Check sheet for the modelled part. Datum: model origin and axes. Units: mm. Face numbers are marked on the shaded views. Give positions to 0.01 mm unless a question says otherwise; leave off trailing zeros. Order: outer loops, then holes, each group sorted by start corner. A loop starts at its lowest first (then second) coordinate and runs counter-clockwise, first axis right, second up.
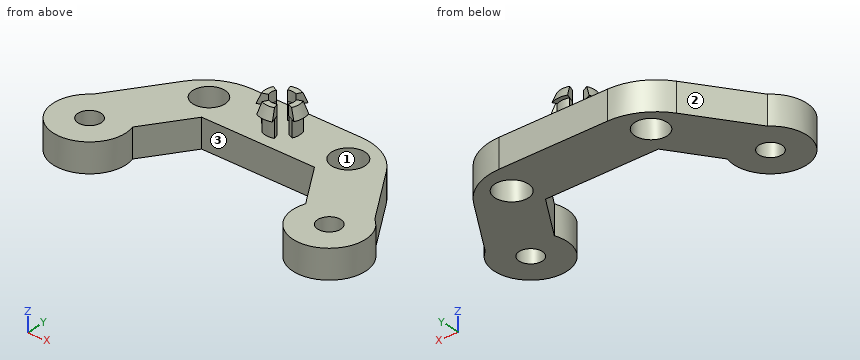
```python
from build123d import *

# Parameters (mm, degrees)
SZKIC1_R                    = 2
DODANIE_WYCI_GNI_CIE1_DEPTH = 5
SZKIC2_R                    = 2.797439786
SZKIC2_R_2                  = 2.890763472
WYTNIJ_WYCI_GNI_CIE1_DEPTH  = 10
ZAOKR_GLENIE1_R             = 10
DODANIE_WYCI_GNI_CIE2_DEPTH = 3
OBR_T1_ANGLE                = 45
SZYK_KO_OWY1_COUNT          = 4


# Read off the part's stored shape, not the designer's step: Obrót1
with BuildPart() as part:
    # Szkic1 → Dodanie-wyciągnięcie1 (new body)
    with BuildSketch(Plane.XY):
        with BuildLine():
            Line((-15, 0), (15, 0))
            Line((15, 0), (25, -15))
            ThreePointArc((25, -15), (23.099320571, -25.970135126), (15.330219835, -17.995329753))
            Line((15.330219835, -17.995329753), (10, -10))
            Line((10, -10), (-10, -10))
            Line((-10, -10), (-15.330219835, -17.995329753))
            ThreePointArc((-15.330219835, -17.995329753), (-23.099320571, -25.970135126), (-25, -15))
            Line((-25, -15), (-15, 0))
        make_face()
        with Locations((-21.25, -20)):
            Circle(SZKIC1_R, mode=Mode.SUBTRACT)
        with Locations((21.25, -20)):
            Circle(SZKIC1_R, mode=Mode.SUBTRACT)
    extrude(amount=DODANIE_WYCI_GNI_CIE1_DEPTH)

    # Szkic2 → Wytnij-wyciągnięcie1 (cut)
    with BuildSketch(Plane.XY.offset(5)):
        with Locations((-12.676758493, -5.398654495)):
            Circle(SZKIC2_R)
        with Locations((12.029040905, -5.398654495)):
            Circle(SZKIC2_R_2)
    extrude(amount=-WYTNIJ_WYCI_GNI_CIE1_DEPTH, mode=Mode.SUBTRACT)

    # Zaokrąglenie1
    zaokr_glenie1_edges = [part.edges().sort_by_distance(p)[0] for p in [
        (-15, 0, 2.5),
        (15, 0, 2.5),
    ]]
    fillet(zaokr_glenie1_edges, radius=ZAOKR_GLENIE1_R)

    # Szkic3 → Dodanie-wyciągnięcie2 (add)
    with BuildSketch(Plane.XY.offset(5)):
        with BuildLine():
            Line((-0.67948159, -3.118961784), (-1.019222385, -2.178442676))
            ThreePointArc((-1.019222385, -2.178442676), (0.136924764, -2.003126361), (1.272268294, -2.283139056))
            Line((1.272268294, -2.283139056), (0.848178863, -3.188759371))
            ThreePointArc((0.848178863, -3.188759371), (0.091283176, -3.002084241), (-0.67948159, -3.118961784))
        make_face()
        with BuildLine():
            Line((1.870588598, -4.292258312), (2.805882897, -3.938387468))
            ThreePointArc((2.805882897, -3.938387468), (2.999104941, -5.073277223), (2.750688951, -6.197376422))
            Line((2.750688951, -6.197376422), (1.833792634, -5.798250948))
            ThreePointArc((1.833792634, -5.798250948), (1.999403294, -5.048851482), (1.870588598, -4.292258312))
        make_face()
        with BuildLine():
            Line((0.692421598, -6.876313495), (1.038632398, -7.814470242))
            ThreePointArc((1.038632398, -7.814470242), (-0.113665121, -7.997845933), (-1.248768691, -7.727742062))
            Line((-1.248768691, -7.727742062), (-0.832512461, -6.818494708))
            ThreePointArc((-0.832512461, -6.818494708), (-0.075776747, -6.998563956), (0.692421598, -6.876313495))
        make_face()
        with BuildLine():
            Line((-1.884973157, -5.668487992), (-2.827459736, -6.002731988))
            ThreePointArc((-2.827459736, -6.002731988), (-2.996499858, -4.855125566), (-2.717538259, -3.72917908))
            Line((-2.717538259, -3.72917908), (-1.811692173, -4.152786053))
            ThreePointArc((-1.811692173, -4.152786053), (-1.997666572, -4.903417044), (-1.884973157, -5.668487992))
        make_face()
    extrude(amount=DODANIE_WYCI_GNI_CIE2_DEPTH)

    # Obrót1 outline → Obrót1 (revolve)
    with BuildSketch(Plane(origin=(0, -5, 0), x_dir=(0.42261826174070005, 0.9063077870366497, 0), z_dir=(0.9063077870366497, -0.42261826174070005, 0))):
        Polygon((3, 9.8), (2, 9.8), (2, 8), (3.781968342, 8), align=None)
    obr_t1 = revolve(axis=Axis((0, -5, 0), (0, 0, 1)), revolution_arc=OBR_T1_ANGLE)

    # Szyk kołowy1: Obrót1 ×4 about axis
    szyk_ko_owy1_axis = Axis((0, -5, 5), (0, 0, 1))
    for i in range(1, SZYK_KO_OWY1_COUNT):
        add(obr_t1.rotate(szyk_ko_owy1_axis, i * 360 / SZYK_KO_OWY1_COUNT))


solid = part.part
```
(1) Gauge pin test, flat ends, axial feed: pin 1 Ø10 at (x, y) = (18, -5.5) entering from +Z; pin 2 Ø4.5 at (x, y) = (12.03, -5.4) entering from -Z; pin 3 Ø1.5 at (y, z) = (-12, 3.5) entering from +X; pin 4 Ø5.5 at (x, z) = (2, 1.5) entering from -Y. Record the tip position at first contact, or that the pin passes through.
Response values:
pin 1: stops at z = 5
pin 2: passes through
pin 3: stops at x = 23.5
pin 4: stops at y = -10
(2) Cross-section at D-D on z = 2.5. Enter the section's corners in (x, y), then the cut area to 3 significant figures.
Response values:
outline: (-25, -15) arc R6.25 ccw (long way) to (-15.33, -18) - (-10, -10) - (10, -10) - (15.33, -18) arc R6.25 ccw (long way) to (25, -15) - (17.97, -4.45) arc R10 ccw to (9.65, 0) - (-9.65, 0) arc R10 ccw to (-17.97, -4.45) - close; hole circle Ø4 at (-21.25, -20); hole circle Ø5.59 at (-12.68, -5.4); hole circle Ø5.78 at (12.03, -5.4); hole circle Ø4 at (21.25, -20)
area: 642 mm2
(3) Cross-section at A-A on y = -20. Enter the section's corners in (x, z).
Response values:
outline: (-27.5, 0) - (-23.25, 0) - (-23.25, 5) - (-27.5, 5) - close; (-19.25, 0) - (-15, 0) - (-15, 5) - (-19.25, 5) - close; (15, 0) - (19.25, 0) - (19.25, 5) - (15, 5) - close; (23.25, 0) - (27.5, 0) - (27.5, 5) - (23.25, 5) - close
(4) Cross-section at B-B on x = 21. Enter the section's corners in (y, z) (3 decimals), then the cut area to 3 significant figures.
Response values:
outline: (-26.245, 0) - (-21.984, 0) - (-21.984, 5) - (-26.245, 5) - close; (-18.016, 0) - (-9, 0) - (-9, 5) - (-18.016, 5) - close
area: 66.4 mm2
(5) Release check for a two-part mould opening along Y. For the marked faces 1, 2 and 3 record: released by +Y, released by -Y, zero draft, split by the parting line, or undercut.
Response values:
face 1: undercut
face 2: released by +Y
face 3: released by -Y
(6) Cross-section at C-C on z = 9. Enter the section's corners in (x, y), then the cut area to 3 significant figures.
Response values:
outline: (-3.15, -6.14) - (-1.88, -5.68) arc R2 cw to (-1.81, -4.15) - (-3.03, -3.59) arc R3.35 ccw to start; (-1.41, -8.03) arc R3.35 ccw to (1.14, -8.15) - (0.68, -6.88) arc R2 cw to (-0.85, -6.81) - close; (-1.14, -1.85) - (-0.68, -3.12) arc R2 cw to (0.85, -3.19) - (1.41, -1.97) arc R3.35 ccw to start; (1.81, -5.85) - (3.03, -6.41) arc R3.35 ccw to (3.15, -3.86) - (1.88, -4.32) arc R2 cw to start
area: 11.3 mm2
(7) Material ranges on L1, parallel to Y at x = -8, z = 1; L2, parallel to Z at x = 18, y = -20.25; L3, parallel to X at y = -3.5, z = 4.75, recorded low to high.
Response values:
L1: y = -10 to 0
L2: z = 0 to 5
L3: x = -17.25 to -14.73, -10.62 to 9.85, 14.21 to 17.25
